Part model, mm, in its own coordinate system. Give positions to 0.01 mm unless a question says otherwise; leave off trailing zeros. Write each loop counter-clockwise with the first axis right and the second up, starting at its lowest first coordinate (ties: lowest second). Pieces come first, ordered by that corner, then holes. Notation, with made-up numbers: M -8,34.5 L 5,34.5 A24 ccw 5,69.5 Z; hole C 59.25,36.25 d8. An arc over 180 degrees is marked long. Use CSV: the item, a comma, the result in double quotes. Start each with the question number.
1. Band-saw the part on B-B, the plane y = 1.15. List the corners of the cut face in (x, z).
2. Drill centre lines: line 1 along X through (y, z) = (1.2, -3.5); line 2 along Z through (x, y) = (47, 0.4); line 3 along X through (y, z) = (0.7, -25). Where is each one in solid material? Low to high. Write a range as from..to.
3. Band-saw the part on C-C, the plane z = 2. List the corners of the cut face in (x, y).
4. Band-saw the part on A-A, the plane x = 57. List the corners of the cut face in (y, z).
Autodesk Fusion 360 part; units mm, degrees
sketch "Sketch1" plane through (0, 0, 0) normal (0, 1, 0) x (1, 0, 0)
  line L0 (70.5, 18) -> (-70.5, 18)
  line L1 (-70.5, 18) -> (-70.5, -18)
  line L2 (-70.5, -18) -> (70.5, -18)
  line L3 (70.5, -18) -> (70.5, 18)
  line L4 (70.5, 18) -> (-70.5, -18) construction
  line L5 (-70.5, 18) -> (70.5, -18) construction
  line L6 (80, 27.5) -> (-80, 27.5)
  line L7 (-80, 27.5) -> (-80, -27.5)
  line L8 (-80, -27.5) -> (80, -27.5)
  line L9 (80, -27.5) -> (80, 27.5)
  line L10 (80, 27.5) -> (-80, -27.5) construction
  line L11 (-80, 27.5) -> (80, -27.5) construction
  dimension "d1" = 141
  dimension "d2" = 36
  dimension "d3" = 160
  dimension "d4" = 55
extrude "Extrude1" add sketch "Sketch1" along normal blind 2
fillet "Fillet1" radius 5 1 edges at (-80, 1, 27.5)
fillet "Fillet2" radius 5 1 edges at (80, 1, 27.5)
fillet "Fillet3" radius 5 1 edges at (80, 1, -27.5)
fillet "Fillet4" radius 5 1 edges at (-80, 1, -27.5)
Output:
1,outline,"M -80,-22.5 A5 ccw -75,-27.5 L 75,-27.5 A5 ccw 80,-22.5 L 80,22.5 A5 ccw 75,27.5 L -75,27.5 A5 ccw -80,22.5 Z; hole M -70.5,-18 L 70.5,-18 L 70.5,18 L -70.5,18 Z"
2,line 1,"x = -80..-70.5, 70.5..80"
2,line 2,"z = -27.5..-18, 18..27.5"
2,line 3,"x = -79.33..79.33"
3,outline,"M -80,0 L -70.5,0 L -70.5,2 L -80,2 Z; M 70.5,0 L 80,0 L 80,2 L 70.5,2 Z"
4,outline,"M 0,-27.5 L 2,-27.5 L 2,-18 L 0,-18 Z; M 0,18 L 2,18 L 2,27.5 L 0,27.5 Z"
